CAD build for the part. Positions are in the model's coordinates, mm. Face numbers are marked on the shaded views. A direction names the side the tool comes from. Give positions to 0.01 mm unless a question says otherwise; leave off trailing zeros. Loops run counter-clockwise (first coordinate to the right, second up) from the corner with the lowest first, then second, coordinate; pieces in that order, holes last.
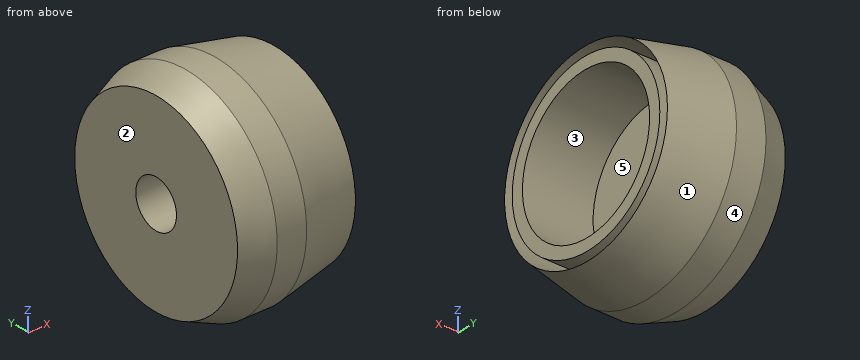
```python
from build123d import *

# Parameters (mm, degrees)
SKETCH022_R      = 9
PAD008_DEPTH     = 10
CHAMFER002_SIZE2 = 1
CHAMFER002_SIZE  = 5
CHAMFER003_SIZE2 = 1
CHAMFER003_SIZE  = 2.5
SKETCH023_R      = 6.25
POCKET014_DEPTH  = 6
SKETCH024_R      = 2
POCKET015_DEPTH  = 5
SKETCH025_R      = 8
SKETCH025_R_2    = 7.25
POCKET016_DEPTH  = 8


with BuildPart() as part:
    # Sketch022 → Pad008 (new body)
    with BuildSketch(Plane.YZ):
        Circle(SKETCH022_R)
    extrude(amount=-PAD008_DEPTH)

    # Chamfer002
    chamfer002_edges = [part.edges().sort_by_distance(p)[0] for p in [
        (0, -9, 0),
    ]]
    chamfer002_side = part.faces().sort_by_distance((-5, -9, 0))[0]
    chamfer(chamfer002_edges, length=CHAMFER002_SIZE, length2=CHAMFER002_SIZE2, reference=chamfer002_side)

    # Chamfer003
    chamfer003_edges = [part.edges().sort_by_distance(p)[0] for p in [
        (-10, -9, 0),
    ]]
    chamfer003_side = part.faces().sort_by_distance((-7.5, -9, 0))[0]
    chamfer(chamfer003_edges, length=CHAMFER003_SIZE, length2=CHAMFER003_SIZE2, reference=chamfer003_side)

    # Sketch023 (on Face5 of Chamfer003) → Pocket014 (cut)
    with BuildSketch(Plane.YZ):
        Circle(SKETCH023_R)
    extrude(amount=-POCKET014_DEPTH, mode=Mode.SUBTRACT)

    # Sketch024 (on Face4 of Pocket014) → Pocket015 (cut)
    with BuildSketch(Plane(origin=(-10, 0, 0), x_dir=(0, 1, 0), z_dir=(-1, 0, 0))):
        Circle(SKETCH024_R)
    extrude(amount=-POCKET015_DEPTH, mode=Mode.SUBTRACT)

    # Sketch025 → Pocket016 (cut)
    with BuildSketch(Plane.YZ):
        Circle(SKETCH025_R)
        Circle(SKETCH025_R_2, mode=Mode.SUBTRACT)
    extrude(amount=-POCKET016_DEPTH, mode=Mode.SUBTRACT)


with BuildPart() as part_1:
    # Body005 placement: moved
    add(part.part.moved(Location((-23, 0, 0))))


solid = part_1.part
```
1. Saw through at B-B, the plane x = -24. List the corners of the cut face in (y, z).
Responses:
outline: circle Ø16.4 at (0, 0); circle Ø14.5 at (0, 0); hole circle Ø16 at (0, 0); hole circle Ø12.5 at (0, 0)
2. Saw through at D-D, the plane x = -28.25. List the corners of the cut face in (y, z), and give its area (3 significant figures).
Responses:
outline: circle Ø18 at (0, 0); circle Ø14.5 at (0, 0); hole circle Ø16 at (0, 0); hole circle Ø12.5 at (0, 0)
area: 95.8 mm2
3. Drop flat-ended pins along their axis: pin 1 (3 mm diameter, centred on x = -32, y = -0.5, fed in from +Z); pin 2 (4 mm diameter, centred on x = -31, z = 5.5, fed in from +Y); pin 3 (4 mm diameter, centred on x = -27, z = 2, fed in from -Y). Give the stop position or say it passes through.
Responses:
pin 1: stops at z = 8.99
pin 2: stops at y = 8.26
pin 3: stops at y = -9
4. Pull direction Z, two halves, no side cores. Call the marked faces 1, 2 and 3: released by +Z, released by -Z, zero draft, split by the parting line, or undercut.
Responses:
face 1: split by the parting line
face 2: zero draft
face 3: undercut
5. Tool access for the marked faces 4 and 5: list every direction of +Z, -Z, +X, -X, +Y, -Y with a clear straight run to the whole face (end or side of a thin tool).
Responses:
face 4: +X, -X
face 5: +X
6. Probe line 1 along Z through (x, y) = (-28.5, 0); line 2 along Z through (x, y) = (-25, 0); line 3 along Y through (x, z) = (-25, 4). List the from-to ranges inside material, lowest first.
Responses:
line 1: z = -9 to -8, -7.25 to -6.25, 6.25 to 7.25, 8 to 9
line 2: z = -8.4 to -8, -7.25 to -6.25, 6.25 to 7.25, 8 to 8.4
line 3: y = -7.39 to -6.93, -6.05 to -4.8, 4.8 to 6.05, 6.93 to 7.39
7. Saw through at A-A, the plane y = 0. List the corners of the cut face in (x, z).
Responses:
outline: (-33, -8) - (-30.5, -9) - (-28, -9) - (-23, -8) - (-31, -8) - (-31, -7.25) - (-23, -7.25) - (-23, -6.25) - (-29, -6.25) - (-29, -2) - (-33, -2) - close; (-33, 2) - (-29, 2) - (-29, 6.25) - (-23, 6.25) - (-23, 7.25) - (-31, 7.25) - (-31, 8) - (-23, 8) - (-28, 9) - (-30.5, 9) - (-33, 8) - close
